Source: three-view drawing plus pictorial views. Frame: mm from the lowest corner of the part. Coordinates: 2 decimals unless noted, no trailing zeros. Order: outer loops, then holes, each group sorted by start corner. A loop starts at its lowest first (then second) coordinate and runs counter-clockwise, first axis right, second up. Notation, with made-up numbers: M 3.25,67 L 45.25,67 A20 cw 45.25,103 Z; hole C -20,-24.5 d5. An arc over 180 degrees is marked long. Use CSV: the item, a comma, the result in double quotes. Start each with the question number.
Q1. Ray query, probe 1 along Y at (x, z) = (26.5, 1.25); probe 2 along X at (y, z) = (2, 0.35). Return the intervals inside material, ascending.
Q2. Section query B-B, the plane x = 32. Output: boundary loops of the cut face in (y, z), and give its area (3 significant figures).
Q3. First-contact query: P1, Ø0.9, axis at y = 2.5, z = 1, coming from the -X side; P2, Ø0.9, axis at x = 67.5, z = 0.5, coming from the +Y side; P3, Ø0.9, axis at x = 64.5, z = 0.5, coming from the -Y side. Flat tips, straight axial feed; report the tip coordinate or a pass-through.
Q4. Section query C-C, the plane y = 28.5. Output: boundary loops of the cut face in (x, z).
Q5. Section query A-A, the plane z = 1.05. Output: boundary loops of the cut face in (x, y), and give its area (3 significant figures).
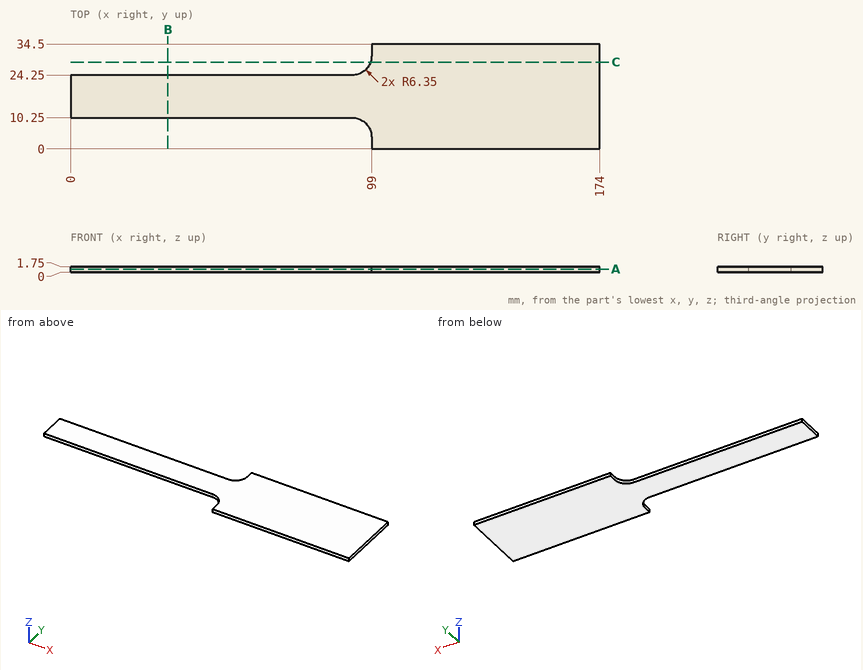
Responses:
1,probe 1,"y = 10.25 to 24.25"
1,probe 2,"x = 99 to 174"
2,outline,"M 10.25,0 L 24.25,0 L 24.25,1.75 L 10.25,1.75 Z"
2,area,"24.5 mm²"
3,P1,"stops at x = 99"
3,P2,"stops at y = 24.25"
3,P3,"stops at y = 10.25"
4,outline,"M 98.64,0 L 174,0 L 174,1.75 L 98.64,1.75 Z"
5,outline,"M 0,10.25 L 92.65,10.25 A6.35 cw 99,3.9 L 99,0 L 174,0 L 174,34.5 L 99,34.5 L 99,30.6 A6.35 cw 92.65,24.25 L 0,24.25 Z"
5,area,"3,990 mm²"
